Geometry check sheet. Reference: drawing and pictorial views, mm from the part's lowest x, y, z. A direction names the side the tool comes from. Coordinates: 2 decimals unless noted, no trailing zeros. Loops run counter-clockwise (first coordinate to the right, second up) from the corner with the lowest first, then second, coordinate; pieces in that order, holes last. Notation, with made-up numbers: (78, 51) - (105, 51) arc R11 cw to (105, 64) - close; hole circle Ø9 at (10, -35). An arc over 180 degrees is marked (long way). Write each question's results on one line, items separated by ' | '. Start each with the question number.
1. Tool access check on the marked faces 1, 2, 3, 4 and 5. Record the directions out of +Z, -Z, +X, -X, +Y, -Y that give a thin tool (end or side, any length) a straight path to the whole face; none if there is none.
2. Cross-section at C-C (x = 69). Record the cut outline in (y, z), and give its area (3 significant figures).
3. Gauge pin test, flat ends, axial feed: P1, Ø1.5, axis at x = 70, z = 3.5, coming from the +Y side; P2, Ø4, axis at x = 68.5, z = 3, coming from the -Y side; P3, Ø10, axis at x = 45, z = 14.5, coming from the -Y side; P4, Ø1.5, axis at y = 30, z = 2.5, coming from the -X side. Record the tip position at first contact, or that the pin passes through.
4. Cross-section at A-A (y = 14). Record the cut outline in (x, z).
5. Cross-section at D-D (y = 6). Record the cut outline in (x, z).
6. Thickness scan on line 1 (X direction, y = 21.5, z = 8); line 2 (Y direction, x = 4.5, z = 1.5). Record the ranges inside material, lowest first. Write a range as [from, to].
7. Cross-section at B-B (z = 3.5). Record the cut outline in (x, y).
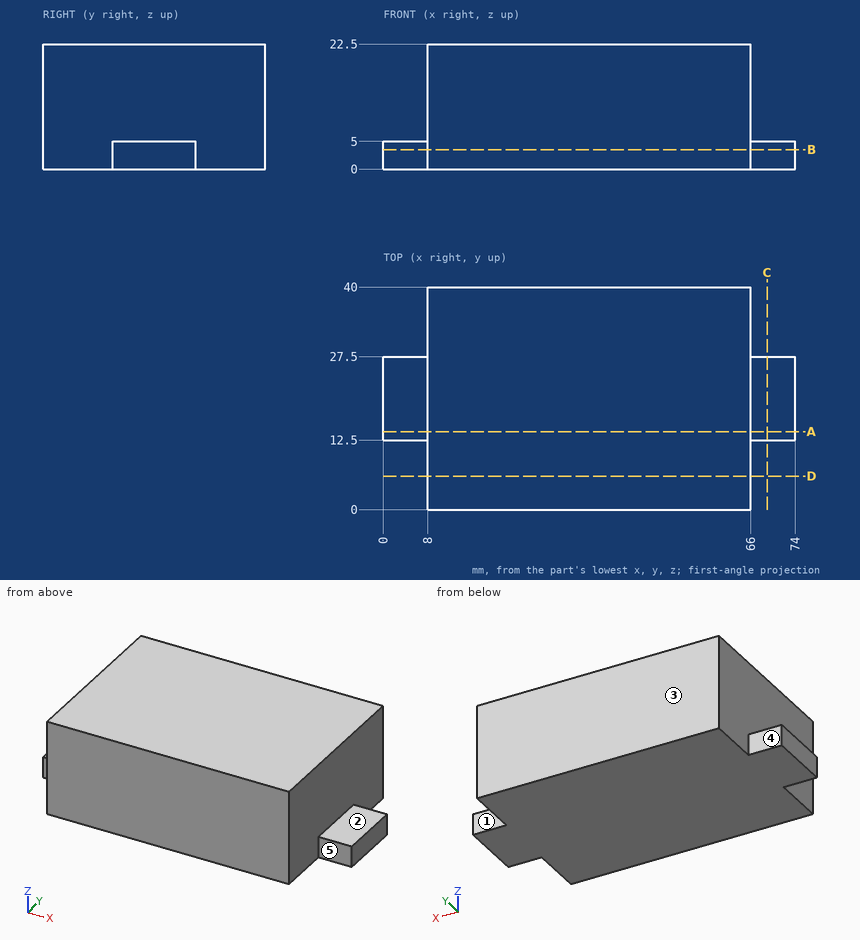
Established:
1) face 1: +Z, -Z, +X, +Y | face 2: +Z, +X, +Y, -Y | face 3: +Z, -Z, +X, -X, +Y | face 4: +Z, -Z, -X, +Y | face 5: +Z, -Z, +X, -Y
2) outline: (12.5, 0) - (27.5, 0) - (27.5, 5) - (12.5, 5) - close | area: 75.0 mm^2
3) P1: y = 27.5 | P2: y = 12.5 | P3: y = 0 | P4: x = 8
4) outline: (0, 0) - (74, 0) - (74, 5) - (66, 5) - (66, 22.5) - (8, 22.5) - (8, 5) - (0, 5) - close
5) outline: (8, 0) - (66, 0) - (66, 22.5) - (8, 22.5) - close
6) line 1: [8, 66] | line 2: [12.5, 27.5]
7) outline: (0, 12.5) - (8, 12.5) - (8, 0) - (66, 0) - (66, 12.5) - (74, 12.5) - (74, 27.5) - (66, 27.5) - (66, 40) - (8, 40) - (8, 27.5) - (0, 27.5) - close
